```python
from build123d import *

# Parameters (mm, degrees)
SKETCH1_R             = 49
SKETCH1_R_2           = 9.9
SKETCH1_W             = 3
SKETCH1_H             = 9
SKETCH1_W_2           = 1
BOSS_EXTRUDE1_DEPTH   = 2.5
BOSS_EXTRUDE2_START   = -5
BOSS_EXTRUDE2_DEPTH   = 5
BOSS_EXTRUDE2_2_DEPTH = 5
BOSS_EXTRUDE2_3_DEPTH = 5
BOSS_EXTRUDE2_4_DEPTH = 5
FILLET1_R             = 0.5
BOSS_EXTRUDE4_DEPTH   = 2.5


with BuildPart() as part:
    # Sketch1 → Boss-Extrude1 (new body)
    with BuildSketch(Plane.XY):
        Circle(SKETCH1_R)
        Circle(SKETCH1_R_2, mode=Mode.SUBTRACT)
        with Locations((0, 40)):
            Rectangle(SKETCH1_W, SKETCH1_H, mode=Mode.SUBTRACT)
        with Locations((-3, 40)):
            Rectangle(SKETCH1_W_2, SKETCH1_H, mode=Mode.SUBTRACT)
    extrude(amount=BOSS_EXTRUDE1_DEPTH)

    # Fillet1
    fillet1_edges = [part.edges().sort_by_distance(p)[0] for p in [
        (0, 35.5, 2.5),
        (0, 44.5, 2.5),
        (-3, 44.5, 2.5),
        (-2.5, 40, 2.5),
        (-3, 35.5, 2.5),
        (-3.5, 40, 2.5),
        (1.5, 40, 2.5),
    ]]
    fillet(fillet1_edges, radius=FILLET1_R)



with BuildPart() as body_2:
    # Sketch1_3 → Boss-Extrude2 (new body)
    with BuildSketch(Plane.XY.offset(BOSS_EXTRUDE2_START)):
        with BuildLine():
            ThreePointArc((9.652460826, 2.2), (7.000357134, 7.000357134), (2.2, 9.652460826))
            Line((2.2, 9.652460826), (2.2, 2.2))
            Line((2.2, 2.2), (9.652460826, 2.2))
        make_face()
    extrude(amount=BOSS_EXTRUDE2_DEPTH)


with BuildPart() as body_3:
    # Sketch1_3 → Boss-Extrude2 2 (new body)
    with BuildSketch(Plane.XY.offset(BOSS_EXTRUDE2_START)):
        with BuildLine():
            Line((-2.2, 2.2), (-2.2, 9.652460826))
            ThreePointArc((-2.2, 9.652460826), (-7.000357134, 7.000357134), (-9.652460826, 2.2))
            Line((-9.652460826, 2.2), (-2.2, 2.2))
        make_face()
    extrude(amount=BOSS_EXTRUDE2_2_DEPTH)


with BuildPart() as body_4:
    # Sketch1_3 → Boss-Extrude2 3 (new body)
    with BuildSketch(Plane.XY.offset(BOSS_EXTRUDE2_START)):
        with BuildLine():
            Line((-2.2, -9.652460826), (-2.2, -2.2))
            Line((-2.2, -2.2), (-9.652460826, -2.2))
            ThreePointArc((-9.652460826, -2.2), (-7.000357134, -7.000357134), (-2.2, -9.652460826))
        make_face()
    extrude(amount=BOSS_EXTRUDE2_3_DEPTH)


with BuildPart() as body_5:
    # Sketch1_3 → Boss-Extrude2 4 (new body)
    with BuildSketch(Plane.XY.offset(BOSS_EXTRUDE2_START)):
        with BuildLine():
            Line((9.652460826, -2.2), (2.2, -2.2))
            Line((2.2, -2.2), (2.2, -9.652460826))
            ThreePointArc((2.2, -9.652460826), (7.000357134, -7.000357134), (9.652460826, -2.2))
        make_face()
    extrude(amount=BOSS_EXTRUDE2_4_DEPTH)


with BuildPart() as part_1:
    add(part.part)

    add(body_2.part)  # Boss-Extrude4 merges body 2

    add(body_3.part)  # Boss-Extrude4 merges body 3

    add(body_4.part)  # Boss-Extrude4 merges body 4

    add(body_5.part)  # Boss-Extrude4 merges body 5
    # Sketch3 → Boss-Extrude4 (add)
    with BuildSketch(Plane.XY):
        with BuildLine():
            Line((-2.2, 2.2), (-2.2, 9.652460826))
            ThreePointArc((-2.2, 9.652460826), (-7.000357134, 7.000357134), (-9.652460826, 2.2))
            Line((-9.652460826, 2.2), (-2.2, 2.2))
        make_face()
        with BuildLine():
            Line((-2.2, -2.2), (-9.652460826, -2.2))
            ThreePointArc((-9.652460826, -2.2), (-7.000357134, -7.000357134), (-2.2, -9.652460826))
            Line((-2.2, -9.652460826), (-2.2, -2.2))
        make_face()
        with BuildLine():
            Line((2.2, -2.2), (2.2, -9.652460826))
            ThreePointArc((2.2, -9.652460826), (7.000357134, -7.000357134), (9.652460826, -2.2))
            Line((9.652460826, -2.2), (2.2, -2.2))
        make_face()
        with BuildLine():
            Line((2.2, 2.2), (9.652460826, 2.2))
            ThreePointArc((9.652460826, 2.2), (7.000357134, 7.000357134), (2.2, 9.652460826))
            Line((2.2, 9.652460826), (2.2, 2.2))
        make_face()
    extrude(amount=BOSS_EXTRUDE4_DEPTH)


solid = part_1.part
```
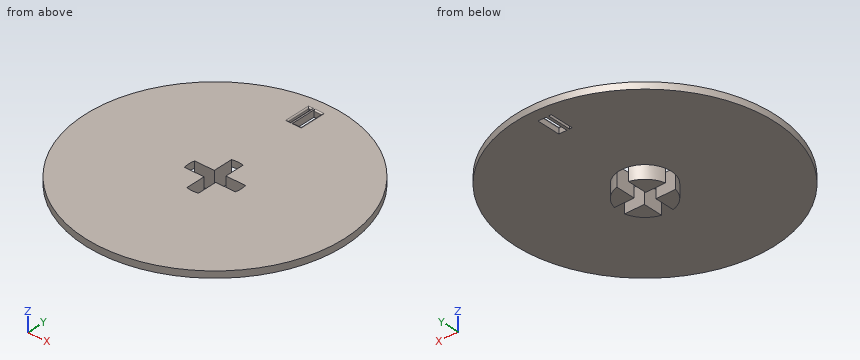
The listing builds one solid part. Answer for the finished solid, in the listing's coordinates (mm). Give positions to 0.01 mm unless a question says otherwise; leave off trailing zeros. Write each loop counter-clockwise with the first axis right and the second up, starting at its lowest first coordinate (ties: lowest second). Pieces come first, ordered by that corner, then holes. Notation, with made-up numbers: (73, -29) -> (88, -29) arc R28 ccw to (88, 10) -> close; hole circle Ø2 at (-13, 4.5). An arc over 180 degrees is marked (long way). Write item = value, one per line. Start each with the question number.
1) The part is cut by section C-C, the plane z = -2.25. Determine the outline of the cut face in (x, y), and give its area (3 significant figures).
2) The part is cut by section B-B, the plane y = 0. Determine the outline of the cut face in (x, z).
3) Each of these flat-tipped pins is pushed along its axis until it touches: pin 1 (1 mm diameter, centred on x = -0.5, z = 1, fed in from +Y); pin 2 (3 mm diameter, centred on x = 16, z = 0, fed in from +Y); pin 3 (2 mm diameter, centred on y = -7.5, z = -3, fed in from +X). Where does it stop, or does it pass through?
4) The part is cut by section A-A, the plane x = 0. Determine the outline of the cut face in (y, z), and give its area (3 significant figures).
5) Straight lines are drawn through the part: line 1 along Z through (x, y) = (19.5, 43); line 2 along Y through (x, z) = (4.5, 0.75); line 3 along Y through (x, z) = (5, 2.25). For each, find the intervals that lie inside material, in ascending order.
6) The part is cut by section D-D, the plane x = 24. Determine the outline of the cut face in (y, z), and give its area (3 significant figures).
Solutions:
q1.outline = (-9.65, -2.2) arc R9.9 ccw to (-2.2, -9.65) -> (-2.2, -2.2) -> close; (-9.65, 2.2) -> (-2.2, 2.2) -> (-2.2, 9.65) arc R9.9 ccw to start; (2.2, -9.65) arc R9.9 ccw to (9.65, -2.2) -> (2.2, -2.2) -> close; (2.2, 2.2) -> (9.65, 2.2) arc R9.9 ccw to (2.2, 9.65) -> close
q1.area = 154 mm²
q2.outline = (-49, 0) -> (-9.9, 0) -> (-9.9, 2.5) -> (-49, 2.5) -> close; (9.9, 0) -> (49, 0) -> (49, 2.5) -> (9.9, 2.5) -> close
q3.pin_1 = 49
q3.pin_2 = 46.81
q3.pin_3 = 7.47
q4.outline = (-49, 0) -> (-9.9, 0) -> (-9.9, 2.5) -> (-49, 2.5) -> close; (9.9, 0) -> (35.5, 0) -> (35.5, 2) arc R0.5 ccw to (35, 2.5) -> (9.9, 2.5) -> close; (44.5, 0) -> (49, 0) -> (49, 2.5) -> (45, 2.5) arc R0.5 ccw to (44.5, 2) -> close
q4.area = 173 mm²
q5.line_1 = 0 to 2.5
q5.line_2 = -48.79 to -2.2, 2.2 to 48.79
q5.line_3 = -48.74 to -2.2, 2.2 to 48.74
q6.outline = (-42.72, 0) -> (42.72, 0) -> (42.72, 2.5) -> (-42.72, 2.5) -> close
q6.area = 214 mm²
